Answer from the drawing. Dimensions are ordinates in mm from the lowest x, y and z of the part. A direction names the side the tool comes from. Coordinates: 2 decimals unless noted, no trailing zeros. Write each loop counter-clockwise with the first axis right and the second up, starting at its lowest first coordinate (ties: lowest second). Pieces come first, ordered by that corner, then holes.
1) Each of these flat-tipped pins is pushed along its axis until it touches: pin 1 Ø6 at (x, y) = (6, 8) entering from -Z; pin 2 Ø1.8 at (x, z) = (15, 9.5) entering from +Y; pin 3 Ø3 at (x, z) = (5.55, 10.55) entering from +Y; pin 4 Ø2.5 at (x, y) = (11, 4) entering from +Z. Where does it stop, or does it pass through?
2) Find the intervals of material crossed by line 1 (X direction, y = 5, z = 11.5); line 2 (Y direction, x = 1.25, z = 15); line 3 (Y direction, x = 4.75, z = 15.5), in increasing order.
3) The part is cut by section C-C (y = 9.5). Determine the outline of the cut face in (x, z), then the cut area to 3 significant figures.
4) Determine the mould class of the marked faces 1, 2 and 3 for opening direction X: +X half, -X half, draft (parallel to the pull), parting line (faces both ways), or undercut.
5) Which of the six approach directions +Z, -Z, +X, -X, +Y, -Y give full straight-line access (tool end or side, diameter ignored) to the marked faces 4, 5, 6 and 7?
6) The part is cut by section A-A (x = 10.55). Determine the outline of the cut face in (y, z).
7) The part is cut by section D-D (x = 19.5). Determine the outline of the cut face in (y, z).
8) The part is cut by section B-B (z = 10.55). Determine the outline of the cut face in (x, y).
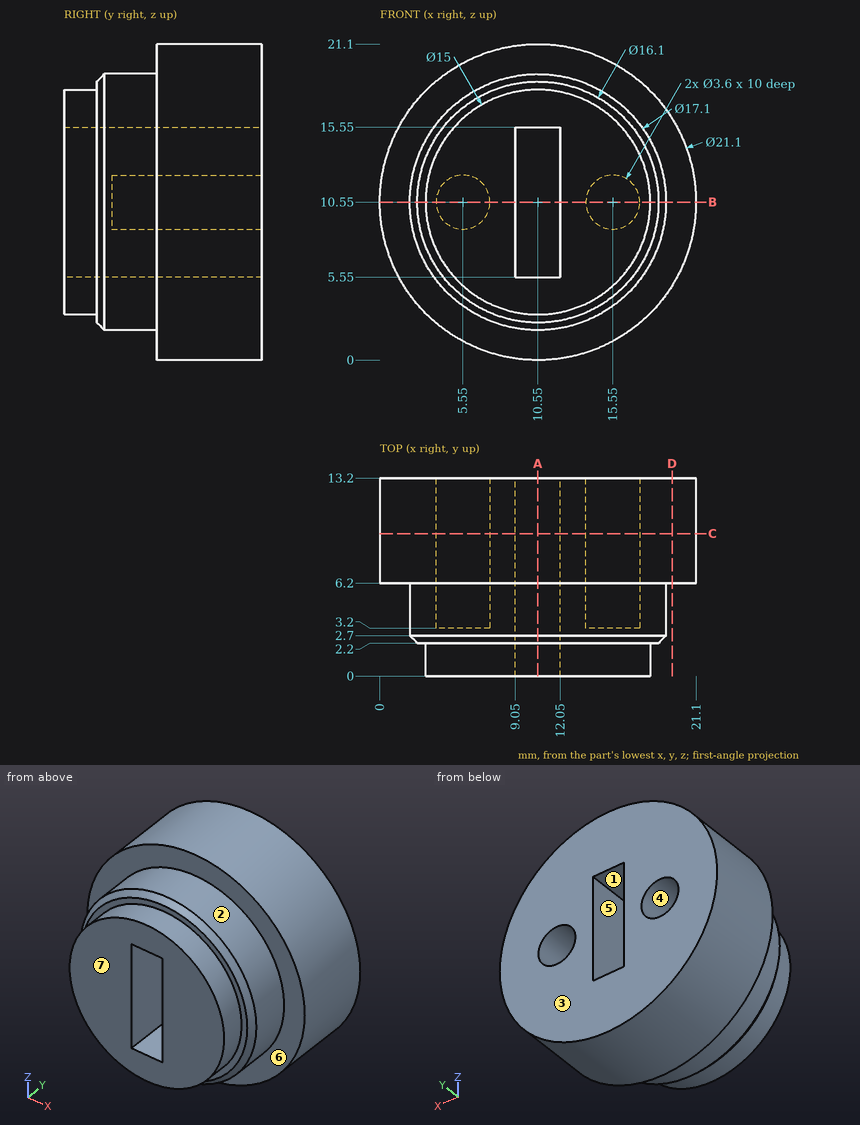
Reported:
1. pin 1: stops at z = 0.11
1. pin 2: stops at y = 13.2
1. pin 3: stops at y = 3.2
1. pin 4: stops at z = 19.1
2. line 1: x = 2.05 to 4.02, 7.08 to 9.05, 12.05 to 14.02, 17.08 to 19.05
2. line 2: y = 6.2 to 13.2
2. line 3: y = 2.2 to 13.2
3. outline: circle Ø21.1 at (10.55, 10.55); hole circle Ø3.6 at (5.55, 10.55); hole (9.05, 5.55) - (12.05, 5.55) - (12.05, 15.55) - (9.05, 15.55) - close; hole circle Ø3.6 at (15.55, 10.55)
3. area: 299 mm2
4. face 1: undercut
4. face 2: parting line
4. face 3: draft
5. face 4: +Y
5. face 5: +Y, -Y
5. face 6: -Y
5. face 7: +Z, -Z, +X, -X, -Y
6. outline: (0, 3.05) - (2.2, 3.05) - (2.2, 2.5) - (2.7, 2) - (6.2, 2) - (6.2, 0) - (13.2, 0) - (13.2, 5.55) - (0, 5.55) - close; (0, 15.55) - (13.2, 15.55) - (13.2, 21.1) - (6.2, 21.1) - (6.2, 19.1) - (2.7, 19.1) - (2.2, 18.6) - (2.2, 18.05) - (0, 18.05) - close
7. outline: (6.2, 4.96) - (13.2, 4.96) - (13.2, 16.14) - (6.2, 16.14) - close
8. outline: (0, 6.2) - (2, 6.2) - (2, 2.7) - (2.5, 2.2) - (3.05, 2.2) - (3.05, 0) - (9.05, 0) - (9.05, 13.2) - (7.35, 13.2) - (7.35, 3.2) - (3.75, 3.2) - (3.75, 13.2) - (0, 13.2) - close; (12.05, 0) - (18.05, 0) - (18.05, 2.2) - (18.6, 2.2) - (19.1, 2.7) - (19.1, 6.2) - (21.1, 6.2) - (21.1, 13.2) - (17.35, 13.2) - (17.35, 3.2) - (13.75, 3.2) - (13.75, 13.2) - (12.05, 13.2) - close
